Here's how the part is built. I have some questions about the finished solid (model axes, mm). Round coordinates to 2 decimals unless told otherwise and drop trailing zeros. Write each loop counter-clockwise with the first axis right and the second up, starting at its lowest first coordinate (ties: lowest second). Pieces come first, ordered by that corner, then holes. Notation, with made-up numbers: (-10, -30.5) - (37, -30.5) arc R20 cw to (37, -19.5) - close; hole circle Ø1 at (85.5, 40.25). An arc over 180 degrees is marked (long way). One line per item, written item: value. Start each with the question number.
Item 1: If I drill on line 1 (Y direction, x = 12, z = -9); line 2 (X direction, y = 107.5, z = 33); line 3 (X direction, y = 119, z = -8), over which ranges is the centre line in solid material (lowest first)?
Item 2: Thinking about a two-plate mould opening in Z: for faces 1 (the face through (1, 101.6, -1)), 2 (the face through (-36.5, 50.8, 12)), 3 (the face through (-23.183, 25.044, -30.235)), which applies, released by +Z, released by -Z, zero draft, split by the parting line, or undercut?
Item 3: Imagine slicing it at A-A, the plane y = 39. Please give me the cut outline in (x, z).
Item 4: For P1, Ø4, axis at x = 16.5, y = 23, coming from the +Z side; P2, Ø5, axis at y = 129.5, z = 30, coming from the -X side; P3, Ø22.5, axis at x = -6.5, z = -10, coming from the +Y side, each with a flat end and sliding along its axis, tell me the tip position at first contact or that it passes through.
```python
from build123d import *

# Parameters (mm, degrees)
SKETCH1_R           = 38.1
BOSS_EXTRUDE1_DEPTH = 50.8
SKETCH2_R           = 41.275
BOSS_EXTRUDE2_DEPTH = 50.8


with BuildPart() as part:
    # Sketch1 → Boss-Extrude1 (new body)
    with BuildSketch(Plane(origin=(0, 0, 0), x_dir=(1, 0, 0), z_dir=(0, 1, 0))):
        with Locations(Location((0, 0, 0), (0, 0, 270))):
            Circle(SKETCH1_R)
    extrude(amount=BOSS_EXTRUDE1_DEPTH)

    # Sketch2 → Boss-Extrude2 (add)
    with BuildSketch(Plane(origin=(0, 50.8, 0), x_dir=(1, 0, 0), z_dir=(0, 1, 0))):
        with Locations(Location((0, 0, 0), (0, 0, 270))):
            Circle(SKETCH2_R)
    extrude(amount=BOSS_EXTRUDE2_DEPTH)

    # Sketch3 → Revolve17 (revolve)
    with BuildSketch(Plane.XY):
        with BuildLine():
            Line((0, 214.429060371), (0, 218.239060371))
            ThreePointArc((0, 218.239060371), (-6.278456146, 216.578582298), (-10.915144585, 212.031350247))
            add(Edge.make_bspline(
                [(-41.275, 101.6), (-41.275, 101.930502855), (-41.273557103, 102.40564964), (-41.268747446, 103.512092248), (-41.257925909, 104.319246857), (-41.246383117, 105.163883335), (-41.228347866, 106.135820012), (-41.200734551, 107.334179726), (-41.159757311, 108.729726347), (-41.100846347, 110.335373987), (-41.029571588, 111.946697142), (-40.946255064, 113.558844584), (-40.850901423, 115.169512919), (-40.743515987, 116.779892998), (-40.624104745, 118.389166096), (-40.459816828, 120.399743968), (-40.238647793, 122.810299788), (-39.945617875, 125.619277994), (-39.562802148, 128.824148418), (-38.809156369, 134.422061303), (-36.96766496, 145.570323281), (-33.49128341, 160.52369707), (-28.30812049, 176.263796505), (-22.487129194, 190.02095936), (-18.428836954, 198.367582764), (-16.193226279, 202.662272388), (-14.657371604, 205.491195217), (-13.781700582, 207.066687496), (-13.19565908, 208.105983946), (-12.707159013, 208.962552916), (-12.311115433, 209.650979413), (-11.92041177, 210.324783551), (-11.526473808, 210.998380475), (-11.168679866, 211.6041541), (-10.999621727, 211.88932335), (-10.915144585, 212.031350247)],
                knots=[0.08301761, 0.08301761, 0.08301761, 0.08301761, 0.08301761, 0.094422695, 0.100125237, 0.105827779, 0.111530322, 0.117232864, 0.128637949, 0.140293389, 0.15194883, 0.163604271, 0.175259711, 0.186915153, 0.198570596, 0.210226038, 0.22188148, 0.245192344, 0.268503208, 0.291814091, 0.315124974, 0.408368487, 0.594855494, 0.734720752, 0.792997941, 0.839619695, 0.862930572, 0.87458601, 0.885991093, 0.891693634, 0.897396175, 0.903098717, 0.908801258, 0.914503799, 0.920206341, 0.920206341, 0.920206341, 0.920206341, 0.920206341], degree=4))
            Line((-41.275, 101.6), (-37.465, 101.6))
            add(Edge.make_bspline(
                [(-37.465, 101.6), (-37.465, 101.930502867), (-37.463557103, 102.405649652), (-37.458747445, 103.51209226), (-37.447925909, 104.31924687), (-37.436383117, 105.163883348), (-37.418347866, 106.135820025), (-37.39073455, 107.334179738), (-37.349757311, 108.729726359), (-37.290846347, 110.335373999), (-37.219571587, 111.946697154), (-37.136255063, 113.558844596), (-37.040901422, 115.169512931), (-36.933515986, 116.779893011), (-36.814104744, 118.389166108), (-36.649816827, 120.39974398), (-36.428647791, 122.8102998), (-36.135617873, 125.619278007), (-35.752802146, 128.82414843), (-34.999156367, 134.422061315), (-33.157664958, 145.570323293), (-29.681283406, 160.523697081), (-24.498120486, 176.263796517), (-18.677129189, 190.020959371), (-14.618836949, 198.367582775), (-12.383226273, 202.662272399), (-10.847371598, 205.491195228), (-9.971700576, 207.066687506), (-9.385659074, 208.105983957), (-8.897159007, 208.962552926), (-8.557849604, 209.552360704), (-8.32017223, 209.962884372), (-8.180293781, 210.203522785), (-8.13830032, 210.275674617)],
                knots=[0.08301761, 0.08301761, 0.08301761, 0.08301761, 0.08301761, 0.094422695, 0.100125237, 0.105827779, 0.111530322, 0.117232864, 0.128637949, 0.140293389, 0.15194883, 0.163604271, 0.175259711, 0.186915153, 0.198570596, 0.210226038, 0.22188148, 0.245192344, 0.268503208, 0.291814091, 0.315124974, 0.408368487, 0.594855494, 0.734720752, 0.792997941, 0.839619695, 0.862930572, 0.87458601, 0.885991093, 0.891693634, 0.897396175, 0.903098717, 0.905533648, 0.905533648, 0.905533648, 0.905533648, 0.905533648], degree=4))
            ThreePointArc((-8.13830032, 210.275674617), (-4.568439157, 213.330693141), (0, 214.429060371))
        make_face()
    revolve(axis=Axis((0, 0, 0), (0, 1, 0)))


solid = part.part
```
Values follow:
1. line 1: y = 0 to 101.6, 197.52 to 204.85
1. line 2: x = -24.66 to -17.57, 17.57 to 24.66
1. line 3: x = -39.78 to -35.88, 35.88 to 39.78
2. face 1: undercut
2. face 2: zero draft
2. face 3: split by the parting line
3. outline: circle Ø76.2 at (0, 0)
4. P1: stops at z = 35.23
4. P2: stops at x = -28.35
4. P3: stops at y = 218.22
